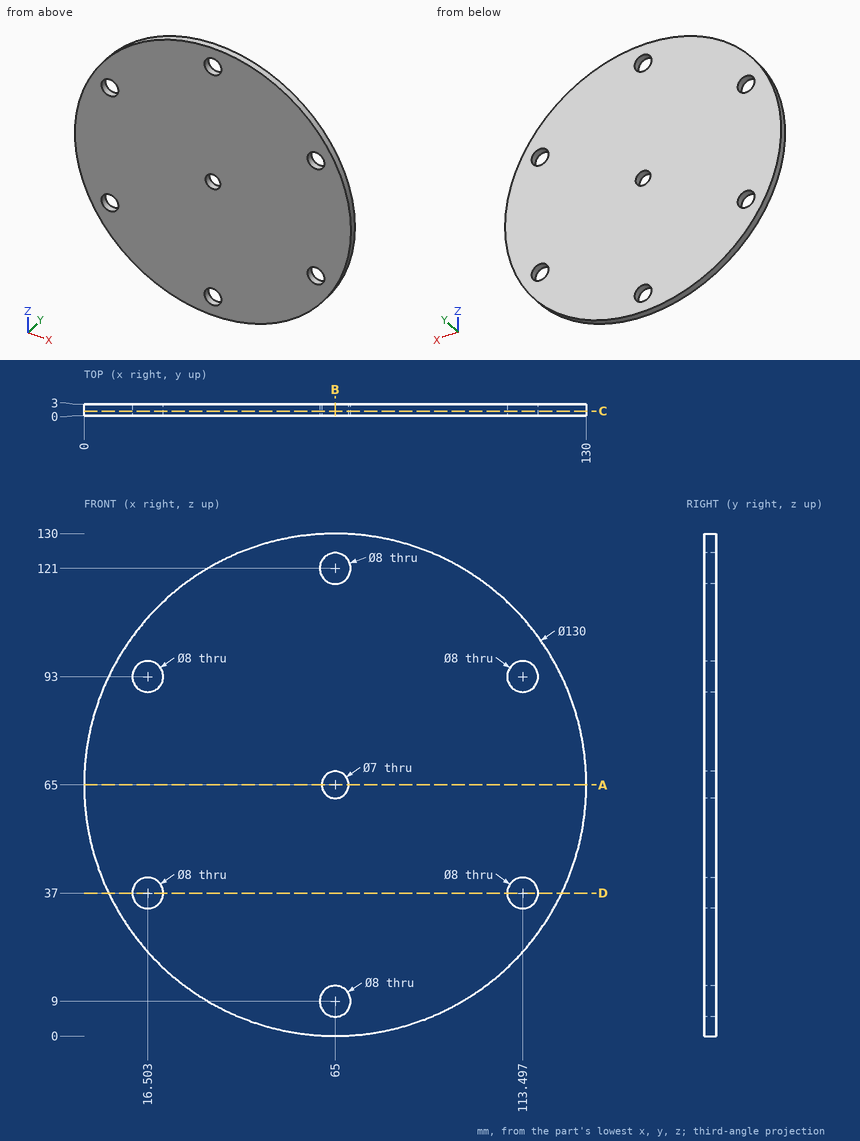
Source: three-view drawing plus pictorial views. Frame: mm from the lowest corner of the part. Coordinates: 2 decimals unless noted, no trailing zeros. Order: outer loops, then holes, each group sorted by start corner. A loop starts at its lowest first (then second) coordinate and runs counter-clockwise, first axis right, second up.
Item 1: Cut plane B-B (x = 65). Return loops of the section in (y, z).
Output values:
outline: (0, 0) - (3, 0) - (3, 5) - (0, 5) - close; (0, 13) - (3, 13) - (3, 61.5) - (0, 61.5) - close; (0, 68.5) - (3, 68.5) - (3, 117) - (0, 117) - close; (0, 125) - (3, 125) - (3, 130) - (0, 130) - close
Item 2: Cut plane C-C (y = 1.15). Return loops of the section in (x, z), plus the area to 3 significant figures.
Output values:
outline: circle Ø130 at (65, 65); hole circle Ø8 at (16.5, 37); hole circle Ø8 at (16.5, 93); hole circle Ø8 at (65, 9); hole circle Ø8 at (65, 121); hole circle Ø7 at (65, 65); hole circle Ø8 at (113.5, 37); hole circle Ø8 at (113.5, 93)
area: 12,900 mm2
Item 3: Cut plane D-D (z = 37). Return loops of the section in (x, y), plus the area to 3 significant figures.
Output values:
outline: (6.34, 0) - (12.5, 0) - (12.5, 3) - (6.34, 3) - close; (20.5, 0) - (109.5, 0) - (109.5, 3) - (20.5, 3) - close; (117.5, 0) - (123.66, 0) - (123.66, 3) - (117.5, 3) - close
area: 304 mm2
Item 4: Cut plane A-A (z = 65). Return loops of the section in (x, y), plus the area to 3 significant figures.
Output values:
outline: (0, 0) - (61.5, 0) - (61.5, 3) - (0, 3) - close; (68.5, 0) - (130, 0) - (130, 3) - (68.5, 3) - close
area: 369 mm2
Item 5: First-contact query: P1, Ø1.5, axis at x = 59.5, y = 1, coming from the +Z side; P2, Ø1, axis at y = 1.5, z = 71.5, coming from the -X side. Flat tips, straight axial feed; report the tip coordinate or a pass-through.
Output values:
P1: stops at z = 129.83
P2: stops at x = 0.28
Item 6: Material intervals for line 1 (Z direction, x = 111, y = 0.85) (1 decimal); line 2 (Z direction, x = 65, y = 1.75); line 3 (Z direction, x = 20, y = 1.3) (1 decimal), sorted ascending.
Output values:
line 1: z = 19.1 to 33.9, 40.1 to 89.9, 96.1 to 110.9
line 2: z = 0 to 5, 13 to 61.5, 68.5 to 117, 125 to 130
line 3: z = 18.1 to 35.1, 38.9 to 91.1, 94.9 to 111.9
